The model under review builds one solid part; all positions refer to its coordinate system, in mm. A direction names the side the tool comes from. Give positions to 0.01 mm unless a question says otherwise; leave off trailing zeros. Order: outer loops, then holes, each group sorted by start corner. A loop starts at its lowest first (then second) coordinate and runs counter-clockwise, first axis right, second up. Notation, with made-up numbers: M 88.25,74 L 106.25,74 A27 ccw 106.25,95 Z; hole C 74,67.25 d3. An arc over 180 degrees is marked long. One line per question, with ' | ' between items. Start each with the question number.
1. We need section D-D on z = 8.5. Write out the cut boundary in (x, y).
2. We need section C-C on x = -18. Write out the cut boundary in (y, z).
3. The part is to be moulded in two halves that separate along Y. For faces 5 (the face through (3, -46, 1)), 6 (the face through (-15.92, -17.35, -10.6)), 7 (the face through (18, -2, -26)), say which applies: +Y half, -Y half, draft (parallel to the pull), parting line (faces both ways), or undercut.
4. For faces 1 (the face through (3, -23, 36)), 2 (the face through (-9, -39.263, 34)), 3 (the face through (-9.47, -8.67, 31.92)), 4 (the face through (13, -39.263, 1)), list the 3-axis set-ups (+Z, -Z, +X, -X, +Y, -Y) from which the entire face can be reached by the end or side of a thin tool; tool diameter is ignored.
5. Insertion check: P1, Ø6, axis at x = -1.5, z = -7.5, coming from the -Y side; P2, Ø5.5, axis at y = -45.5, z = 7.5, coming from the +X side; P3, Ø2, axis at x = -12, z = 47, coming from the +Y side. Each pin has a flat end and moves straight along its axis. Give the tip position at first contact, or say it passes through.
6. Wall thickness on L1, parallel to Y at x = -7.75, z = 43; L2, parallel to X at y = -34.5, z = 39; L3, parallel to X at y = -8.5, z = -21: over which ranges is each line inside the solid? List them lowest first.
7. We need section A-A on x = 15.5. Write out the cut boundary in (y, z), then the cut area to 3 significant figures.
8. We need section B-B on y = -27. Write out the cut boundary in (x, z).
```python
from build123d import *

# Parameters (mm, degrees)
SKETCH1_R               = 7
BOSS_EXTRUDE3_DEPTH     = 22
SKETCH8_R               = 5.5
CUT_EXTRUDE1_DEPTH      = 46
SKETCH10_W              = 34.059077951
SKETCH10_H              = 32.597107019
CUT_EXTRUDE2_DEPTH      = 19
SKETCH19_R              = 41
CUT_EXTRUDE5_DEPTH      = 14
CUT_EXTRUDE5_DEPTH_BACK = 10
SKETCH21_W              = 39.040087977
SKETCH21_H              = 19
CUT_EXTRUDE7_DEPTH      = 19


with BuildPart() as part:
    # Sketch1 → Boss-Extrude3 (new body, symmetric)
    with BuildSketch(Plane(origin=(0, 0, 0), x_dir=(0, 0, -1), z_dir=(1, 0, 0))):
        with BuildLine():
            Line((0, 0), (24, 0))
            Line((24, 0), (29, -5))
            Line((29, -5), (29, -24))
            Line((29, -24), (0, -58))
            Line((0, -58), (-5.703019947, -58))
            ThreePointArc((-5.703019947, -58), (-7.775768892, -55.305839554), (-9.519025669, -52.387647562))
            ThreePointArc((-9.519025669, -52.387647562), (-11.35140658, -48.033040831), (-12.452414435, -43.438696342))
            ThreePointArc((-12.452414435, -43.438696342), (-14.440768413, -40.168970146), (-18.158792561, -39.262903161))
            Line((-18.158792561, -39.262903161), (-50, -39.262903161))
            Line((-50, -39.262903161), (-57, -32.262903161))
            Line((-57, -32.262903161), (-57, -13.71762228))
            Line((-57, -13.71762228), (-50, -6.71762228))
            Line((-50, -6.71762228), (-43, -6.71762228))
            Line((-43, -6.71762228), (-20.519163329, -10.681600334))
            ThreePointArc((-20.519163329, -10.681600334), (-8.446624302, -8.823458857), (0, 0))
        make_face()
        with Locations((-43, -25.262903161)):
            Circle(SKETCH1_R, mode=Mode.SUBTRACT)
    extrude(amount=BOSS_EXTRUDE3_DEPTH, both=True)

    # Sketch8 → Cut-Extrude1 (cut)
    with BuildSketch(Plane(origin=(22, 0, 0), x_dir=(0, 0, -1), z_dir=(1, 0, 0))):
        with Locations((14.962850045, -14)):
            Circle(SKETCH8_R)
    extrude(amount=-CUT_EXTRUDE1_DEPTH, mode=Mode.SUBTRACT)

    # Sketch10 → Cut-Extrude2 (cut)
    with BuildSketch(Plane(origin=(22, 0, 0), x_dir=(0, 0, -1), z_dir=(1, 0, 0))):
        with Locations((-40.029538976, -22.964349652)):
            Rectangle(SKETCH10_W, SKETCH10_H)
    extrude(amount=-CUT_EXTRUDE2_DEPTH, mode=Mode.SUBTRACT)

    # Sketch19 → Cut-Extrude5 (cut, two sides)
    with BuildSketch(Plane(origin=(0, 0, 0), x_dir=(0, 0, -1), z_dir=(1, 0, 0))) as cut_extrude5_sk:
        with Locations((29, 3.701873436)):
            Circle(SKETCH19_R)
    extrude(amount=CUT_EXTRUDE5_DEPTH, mode=Mode.SUBTRACT)
    extrude(cut_extrude5_sk.sketch, amount=-CUT_EXTRUDE5_DEPTH_BACK, mode=Mode.SUBTRACT)

    # Sketch21 → Cut-Extrude7 (cut)
    with BuildSketch(Plane(origin=(22, 0, 0), x_dir=(0, 0, -1), z_dir=(1, 0, 0))):
        with Locations((-3.479956011, -48.762903161)):
            Rectangle(SKETCH21_W, SKETCH21_H)
    extrude(amount=-CUT_EXTRUDE7_DEPTH, mode=Mode.SUBTRACT)


solid = part.part
```
Entries:
1) outline: M -22,-54.19 L 3,-54.19 L 3,-39.26 L 22,-39.26 L 22,-8.85 L 14,-8.85 L 14,-12.87 L -10,-12.87 L -10,-8.85 L -22,-8.85 Z
2) outline: M -58,0 L -24,-29 L -5,-29 L 0,-24 L 0,0 A19 cw -10.68,20.52 L -6.72,43 L -6.72,50 L -13.72,57 L -32.26,57 L -39.26,50 L -39.26,18.16 A5 cw -43.44,12.45 A29 ccw -58,5.7 Z; hole C -25.26,43 d14; hole C -14,-14.96 d11
3) face 5: draft | face 6: undercut | face 7: +Y half
4) face 1: +Z, +X, +Y, -Y | face 2: +Z, +X, -X, -Y | face 3: +X, -X, +Y | face 4: +Z, -Z, +X, -Y
5) P1: stops at y = -52.72 | P2: stops at x = 3 | P3: stops at y = -6.72
6) L1: y = -39.26 to -32.26, -18.26 to -6.72 | L2: x = -22 to 3 | L3: x = -22 to -10, 14 to 22
7) outline: M -39.26,-15.98 L -24,-29 L -5,-29 L 0,-24 L 0,0 A19 cw -10.68,20.52 L -10.24,23 L -39.26,23 L -39.26,18.16 A5 cw -39.26,16.63 Z; hole C -14,-14.96 d11 | area: 1,640 mm^2
8) outline: M -22,-26.44 L -10,-26.44 L -10,-1.83 L 14,-1.83 L 14,-26.44 L 22,-26.44 L 22,23 L 3,23 L 3,36.22 L -22,36.22 Z; M -22,49.78 L 3,49.78 L 3,57 L -22,57 Z
